from build123d import *

# Parameters (mm, degrees)
F0_R     = 8
F1_DEPTH = 1
F2_R     = 6.5
F3_DEPTH = 7
F4_R     = 8
F5_DEPTH = 8
F6_R     = 0.6
F7_DEPTH = 7
F8_R     = 2.5
F9_DEPTH = 16.001
F10_SIZE = 0.25


with BuildPart() as f1:
    # F0 (on Front) → F1 (new body)
    with BuildSketch(Plane.XZ):
        Circle(F0_R)
    extrude(amount=F1_DEPTH)

    # F2 (on face) → F3 (join)
    with BuildSketch(Plane.XZ.offset(1)):
        Circle(F2_R)
    extrude(amount=F3_DEPTH)

    # F4 (on face) → F5 (join)
    with BuildSketch(Plane.XZ.offset(8)):
        Circle(F4_R)
    extrude(amount=F5_DEPTH)

    # F6 (on face) → F7 (cut, through all)
    with BuildSketch(Plane.XZ.offset(1)):
        with Locations((0, 6.5)):
            Circle(F6_R)
        with Locations((-2.00861, 6.181867)):
            Circle(F6_R)
        with Locations((-3.820604, 5.25861)):
            Circle(F6_R)
        with Locations((-5.25861, 3.820604)):
            Circle(F6_R)
        with Locations((-6.181867, 2.00861)):
            Circle(F6_R)
        with Locations((-6.5, 0)):
            Circle(F6_R)
        with Locations((-6.181867, -2.00861)):
            Circle(F6_R)
        with Locations((-5.25861, -3.820604)):
            Circle(F6_R)
        with Locations((-3.820604, -5.25861)):
            Circle(F6_R)
        with Locations((-2.00861, -6.181867)):
            Circle(F6_R)
        with Locations((0, -6.5)):
            Circle(F6_R)
        with Locations((2.00861, -6.181867)):
            Circle(F6_R)
        with Locations((3.820604, -5.25861)):
            Circle(F6_R)
        with Locations((5.25861, -3.820604)):
            Circle(F6_R)
        with Locations((6.181867, -2.00861)):
            Circle(F6_R)
        with Locations((6.5, 0)):
            Circle(F6_R)
        with Locations((6.181867, 2.00861)):
            Circle(F6_R)
        with Locations((5.25861, 3.820604)):
            Circle(F6_R)
        with Locations((3.820604, 5.25861)):
            Circle(F6_R)
        with Locations((2.00861, 6.181867)):
            Circle(F6_R)
    extrude(amount=F7_DEPTH, mode=Mode.SUBTRACT)

    # F8 (on face) → F9 (cut, through all)
    with BuildSketch(Plane.XZ.offset(16)):
        Circle(F8_R)
    extrude(amount=-F9_DEPTH, mode=Mode.SUBTRACT)

    # F10
    f10_edges = [f1.edges().sort_by_distance(p)[0] for p in [
        (8, -12, 0),
        (-8, -8, 0),
        (-8, -16, 0),
        (8, -0.5, 0),
        (-8, 0, 0),
        (-8, -1, 0),
        (-2.5, -16, 0),
        (2.5, -8, 0),
        (-2.5, 0, 0),
    ]]
    chamfer(f10_edges, length=F10_SIZE)


solid = f1.part
Check sheet for the modelled part. Datum: model origin and axes. Units: mm. A direction names the side the tool comes from. Round coordinates to 2 decimals unless told otherwise and drop trailing zeros. Order: outer loops, then holes, each group sorted by start corner. A loop starts at its lowest first (then second) coordinate and runs counter-clockwise, first axis right, second up.
(1) Draft check along Y on faces 4 (the cylindrical face through (4.766, -4.451, 3.478)), 5 (the cylindrical face through (-1.73, -11.95, -7.81)), 6 (the cylindrical face through (5.607, -4.451, 1.835)), 7 (the flat face through (3, 0, 0)). Enter one of: pulls with the +Y half, pulls with the -Y half, needs draft (parallel to the pull), parting line crosses it, or undercut.
(2) Cross-section at A-A, the plane x = 0. Enter the section's corners in (y, z), and give its area (3 significant figures).
(3) Cross-section at B-B, the plane z = 0. Enter the section's corners in (x, y).
(4) Go/stop test with flat-tipped pins: P1, Ø8, axis at y = -4, z = -3.5, coming from the -X side; P2, Ø4, axis at x = -1, y = -4.5, coming from the -Z side; P3, Ø2, axis at y = -11.5, z = 2, coming from the +X side. Record where each tip stops, or that it passes through.
(5) Cross-section at C-C, the plane y = -11. Enter the section's corners in (x, z), and give its area (3 significant figures).
(6) Scan lines: probe 1 along Z at (x, y) = (0, -12.5); probe 2 along Y at (x, z) = (-5.75, -3.25); probe 3 along Z at (x, y) = (0, -6). Record each from-to range of solid material in increasing order.
(7) Access from +Z, -Z, +X, -X, +Y, -Y to the whole of each face (thin tool, end or side, straight path). Record for faces 1 (the cylindrical face through (-4.78, -4.45, 3.46)), 2 (the cylindrical face through (0, -4.5, 5.9)), 3 (the cylindrical face through (6.42, -4.45, -1.02)).
Check sheet entries:
1. face 4: undercut
1. face 5: needs draft
1. face 6: undercut
1. face 7: pulls with the +Y half
2. outline: (-16, -7.75) - (-15.75, -8) - (-8.25, -8) - (-8, -7.75) - (-8, -5.9) - (-1, -5.9) - (-1, -7.75) - (-0.75, -8) - (-0.25, -8) - (0, -7.75) - (0, -2.75) - (-0.25, -2.5) - (-15.75, -2.5) - (-16, -2.75) - close; (-16, 2.75) - (-15.75, 2.5) - (-0.25, 2.5) - (0, 2.75) - (0, 7.75) - (-0.25, 8) - (-0.75, 8) - (-1, 7.75) - (-1, 5.9) - (-8, 5.9) - (-8, 7.75) - (-8.25, 8) - (-15.75, 8) - (-16, 7.75) - close
2. area: 146 mm2
3. outline: (-8, -15.75) - (-7.75, -16) - (-2.75, -16) - (-2.5, -15.75) - (-2.5, -0.25) - (-2.75, 0) - (-7.75, 0) - (-8, -0.25) - (-8, -0.75) - (-7.75, -1) - (-5.9, -1) - (-5.9, -8) - (-7.75, -8) - (-8, -8.25) - close; (2.5, -15.75) - (2.75, -16) - (7.75, -16) - (8, -15.75) - (8, -8.25) - (7.75, -8) - (5.9, -8) - (5.9, -1) - (7.75, -1) - (8, -0.75) - (8, -0.25) - (7.75, 0) - (2.75, 0) - (2.5, -0.25) - close
4. P1: stops at x = -7.91
4. P2: stops at z = -6.47
4. P3: stops at x = 7.94
5. outline: circle Ø16 at (0, 0); hole circle Ø5 at (0, 0)
5. area: 181 mm2
6. probe 1: z = -8 to -2.5, 2.5 to 8
6. probe 2: y = -16 to -8, -1 to 0
6. probe 3: z = -5.9 to -2.5, 2.5 to 5.9
7. face 1: none
7. face 2: +Z
7. face 3: -Z, +X
